Design review of the part built by this model. Coordinates are the model's own, in mm. Face numbers are marked on the shaded views. A direction names the side the tool comes from. Round coordinates to 2 decimals unless told otherwise and drop trailing zeros. Loops run counter-clockwise (first coordinate to the right, second up) from the corner with the lowest first, then second, coordinate; pieces in that order, holes last. Notation, with made-up numbers: M -6,21 L 48,21 A27 ccw 48,43 Z; hole C 5,64.25 d10. An arc over 180 degrees is marked long. One line per item, written item: value. Start each with the question number.
Item 1: We need section C-C (x = 13.75). Write out the cut boundary in (y, z), then the cut area to 3 significant figures.
Item 2: We need section A-A (y = 0). Write out the cut boundary in (x, z).
Item 3: We need section D-D (y = -4). Write out the cut boundary in (x, z), then the cut area to 3 significant figures.
Item 4: Mouldability with a two-part tool opening along X and no side actions: class the marked faces 1, 2 and 3 as released by +X, released by -X, zero draft, split by the parting line, or undercut.
Item 5: For the marked faces 4, 5, 6, 7 and 8, list the 3-axis set-ups (+Z, -Z, +X, -X, +Y, -Y) from which the entire face can be reached by the end or side of a thin tool; tool diameter is ignored.
Item 6: Clearance check with flat-ended pins moving along their axes: pin 1 (10 mm diameter, centred on x = 0, z = 14, fed in from +Y); pin 2 (1.2 mm diameter, centred on x = 13.5, z = 33, fed in from +Y); pin 3 (3 mm diameter, centred on x = 2.5, z = 34, fed in from -Y). State where each tip first meets the part, or that it passes through.
Item 7: For line 1 along X through (y, z) = (7, 32.25); line 2 along Z through (x, y) = (-13.75, 7.75); line 3 along X through (y, z) = (-2.8, 23), list the stretches that pass through material, from the lowest coordinate up.
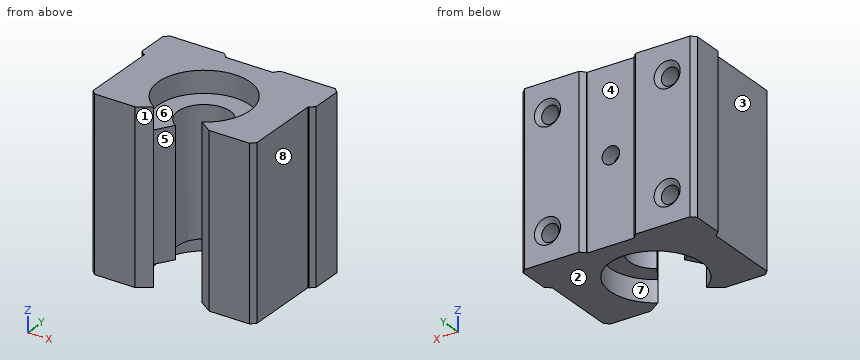
from build123d import *

# Parameters (mm, degrees)
SALIENTE_EXTRUIR1_DEPTH = 39
CORTAR_EXTRUIR1_DEPTH   = 39
SALIENTE_EXTRUIR2_DEPTH = 29
CROQUIS5_R              = 2
CORTAR_EXTRUIR2_DEPTH   = 17
CROQUIS6_R              = 2
CORTAR_EXTRUIR3_DEPTH   = 4
CHAFL_N1_SIZE           = 1


with BuildPart() as part:
    # Croquis1 → Saliente-Extruir1 (new body)
    with BuildSketch(Plane.XY):
        Polygon((-5.5, 13.7), (-5.5, 12.5), (5.5, 12.5), (5.5, 13.7), (20, 13.7), (20, 4.7), (18.8, 4.7), (18.8, -13.7), (-18.8, -13.7), (-18.8, 4.7), (-20, 4.7), (-20, 13.7), align=None)
    extrude(amount=SALIENTE_EXTRUIR1_DEPTH)

    # Croquis2 → Cortar-Extruir1 (cut)
    with BuildSketch(Plane.XY.offset(39)):
        with BuildLine():
            Line((-5.571355311, -11.7), (-8.5, -13.7))
            Line((-8.5, -13.7), (8.5, -13.7))
            Line((8.5, -13.7), (5.571355311, -11.7))
            ThreePointArc((5.571355311, -11.7), (0, 7.7), (-5.571355311, -11.7))
        make_face()
    extrude(amount=-CORTAR_EXTRUIR1_DEPTH, mode=Mode.SUBTRACT)

    # Croquis3 → Saliente-Extruir2 (add)
    with BuildSketch(Plane(origin=(0, 0, 5), x_dir=(-1, 0, 0), z_dir=(0, 0, -1))):
        with BuildLine():
            Line((-3.183631606, -7.885714286), (-5.571355311, -11.7))
            ThreePointArc((-5.571355311, -11.7), (0, 7.7), (5.571355311, -11.7))
            Line((5.571355311, -11.7), (3.183631606, -7.885714286))
            ThreePointArc((3.183631606, -7.885714286), (0, 3.2), (-3.183631606, -7.885714286))
        make_face()
    extrude(amount=-SALIENTE_EXTRUIR2_DEPTH)

    # Croquis5 → Cortar-Extruir2 (cut)
    with BuildSketch(Plane(origin=(0, 13.7, 0), x_dir=(1, 0, 0), z_dir=(0, 1, 0))):
        with Locations((13.75, -32.25)):
            Circle(CROQUIS5_R)
        with Locations((-13.75, -32.25)):
            Circle(CROQUIS5_R)
        with Locations((13.75, -6.75)):
            Circle(CROQUIS5_R)
        with Locations((-13.75, -6.75)):
            Circle(CROQUIS5_R)
    extrude(amount=-CORTAR_EXTRUIR2_DEPTH, mode=Mode.SUBTRACT)

    # Croquis6 → Cortar-Extruir3 (cut)
    with BuildSketch(Plane(origin=(0, 12.5, 0), x_dir=(1, 0, 0), z_dir=(0, 1, 0))):
        with Locations((0, -19.5)):
            Circle(CROQUIS6_R)
    extrude(amount=-CORTAR_EXTRUIR3_DEPTH, mode=Mode.SUBTRACT)

    # Chaflán1
    chafl_n1_edges = [part.edges().sort_by_distance(p)[0] for p in [
        (20, 4.7, 19.5),
        (18.8, -13.7, 19.5),
        (-18.8, -13.7, 19.5),
        (-20, 4.7, 19.5),
        (-20, 13.7, 19.5),
        (-5.5, 13.7, 19.5),
        (5.5, 13.7, 19.5),
        (20, 13.7, 19.5),
        (11.75, 13.7, 32.25),
        (-15.75, 13.7, 32.25),
        (11.75, 13.7, 6.75),
        (-15.75, 13.7, 6.75),
    ]]
    chamfer(chafl_n1_edges, length=CHAFL_N1_SIZE)


solid = part.part
A:
1. outline: M -13.7,0 L 13.7,0 L 13.7,3.75 L 12.7,4.75 L -3.3,4.75 L -3.3,8.75 L 12.7,8.75 L 13.7,9.75 L 13.7,29.25 L 12.7,30.25 L -3.3,30.25 L -3.3,34.25 L 12.7,34.25 L 13.7,35.25 L 13.7,39 L -13.7,39 Z
1. area: 931 mm2
2. outline: M -18.8,0 L -10.12,0 L -10.12,5 L -5.31,5 L -5.31,34 L -10.12,34 L -10.12,39 L -18.8,39 Z; M 5.31,5 L 10.12,5 L 10.12,0 L 18.8,0 L 18.8,39 L 10.12,39 L 10.12,34 L 5.31,34 Z; hole C -13.75,6.75 d4; hole C -13.75,32.25 d4; hole C 13.75,6.75 d4; hole C 13.75,32.25 d4
3. outline: M -18.8,0 L -10.43,0 L -10.43,5 L -5.88,5 L -5.88,34 L -10.43,34 L -10.43,39 L -18.8,39 Z; M 5.88,5 L 10.43,5 L 10.43,0 L 18.8,0 L 18.8,39 L 10.43,39 L 10.43,34 L 5.88,34 Z
3. area: 917 mm2
4. face 1: undercut
4. face 2: zero draft
4. face 3: released by -X
5. face 4: +Z, -Z, +Y
5. face 5: +Z, -Z, -Y
5. face 6: +Z
5. face 7: -Z
5. face 8: +Z, -Z, +X, -Y
6. pin 1: y = 12.5
6. pin 2: y = -3.3
6. pin 3: y = -9.19
7. line 1: -20 to -15.75, -11.75 to 11.75, 15.75 to 20
7. line 2: 0 to 4.75, 8.75 to 30.25, 34.25 to 39
7. line 3: -18.8 to -6, 6 to 18.8
